Source: three-view drawing plus pictorial views. Frame: mm from the lowest corner of the part. A direction names the side the tool comes from. Give positions to 0.01 mm unless a question says otherwise; leave off trailing zeros. Loops run counter-clockwise (first coordinate to the right, second up) from the corner with the lowest first, then second, coordinate; pieces in that order, holes last.
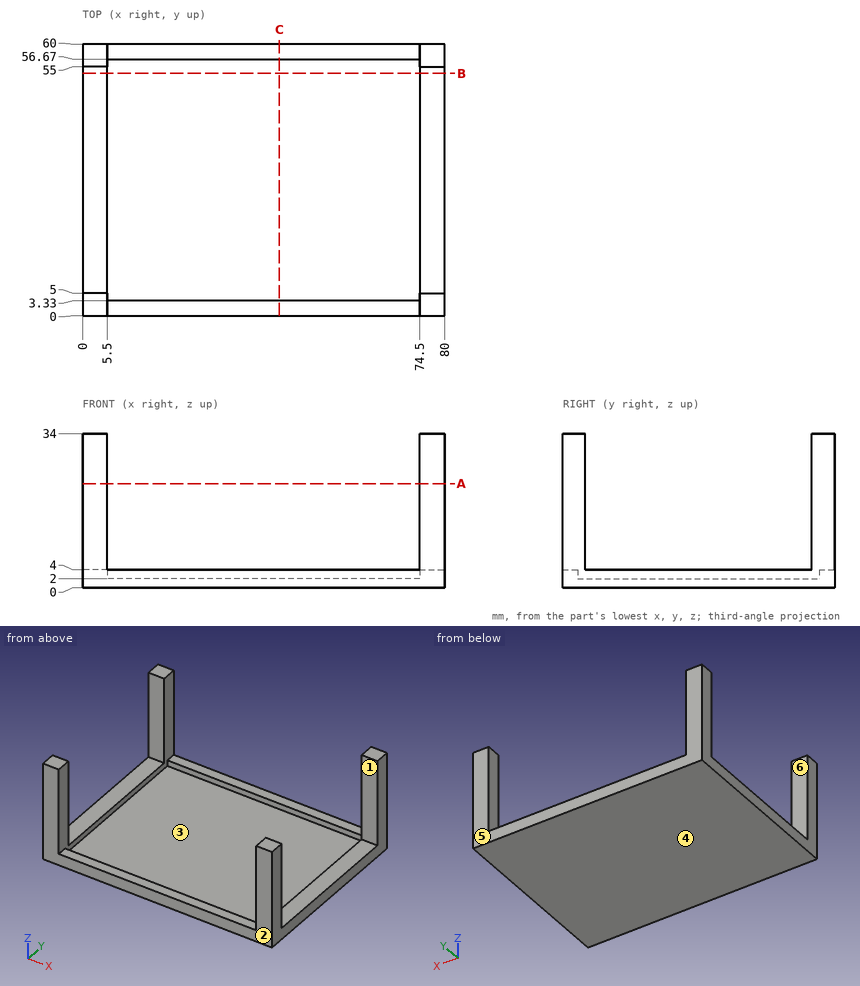
Q1. Section query B-B, the plane y = 53.5. Return loops of the section in (x, z), and give its area (3 significant figures).
Q2. Material intervals for probe 1 along Y at (x, z) = (60, 3); probe 2 along Z at (x, y) = (38, 34); probe 3 along X at (y, z) = (3, 7.5), sorted ascending.
Q3. Section query A-A, the plane z = 23. Return loops of the section in (x, y).
Q4. Reachability of the marked faces 1 and 2 from +Z, -Z, +X, -X, +Y, -Y: full face, straight path, thin tool, end or side. Return the list, or none.
Q5. Pin query (flat end, axial travel): pin 1 Ø1.7 at (x, y) = (47.5, 58.5) entering from +Z; pin 2 Ø5 at (x, y) = (63.5, 38) entering from -Z; pin 3 Ø8 at (x, y) = (40, 40.5) entering from +Z. Return the tip coordinate at first contact, or that it passes through.
Q6. Mould query, pull axis Y, two halves, no side actions, for the marked faces 3, 4, 5 and 6. Classes: +Y half, -Y half, draft (parallel to the pull), parting line (faces both ways), or undercut.
Q7. Section query C-C, the plane x = 43.5. Return loops of the section in (y, z), and give its area (3 significant figures).
Resolved:
1. outline: (0, 0) - (80, 0) - (80, 4) - (74.5, 4) - (74.5, 2) - (5.5, 2) - (5.5, 4) - (0, 4) - close
1. area: 182 mm2
2. probe 1: y = 0 to 3.33, 56.67 to 60
2. probe 2: z = 0 to 2
2. probe 3: x = 0 to 5.5, 74.5 to 80
3. outline: (0, 0) - (5.5, 0) - (5.5, 5) - (0, 5) - close; (0, 55) - (5.5, 55) - (5.5, 60) - (0, 60) - close; (74.5, 0) - (80, 0) - (80, 5) - (74.5, 5) - close; (74.5, 55) - (80, 55) - (80, 60) - (74.5, 60) - close
4. face 1: +Z, +X, -X
4. face 2: +Z, -Z, +X, -X, -Y
5. pin 1: stops at z = 4
5. pin 2: stops at z = 0
5. pin 3: stops at z = 2
6. face 3: undercut
6. face 4: draft
6. face 5: +Y half
6. face 6: undercut
7. outline: (0, 0) - (60, 0) - (60, 4) - (56.67, 4) - (56.67, 2) - (3.33, 2) - (3.33, 4) - (0, 4) - close
7. area: 133 mm2
